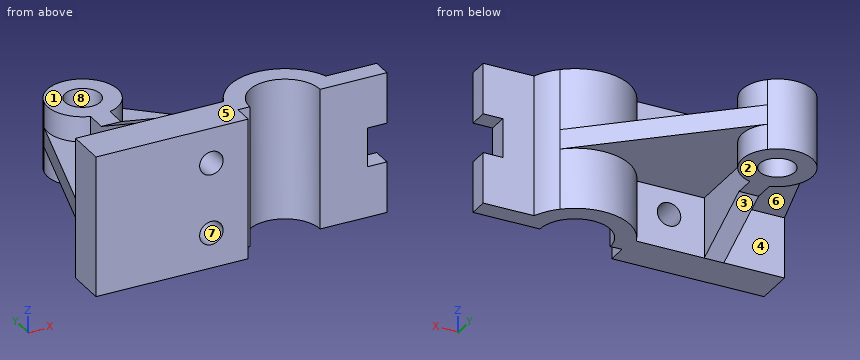
```python
from build123d import *

# Parameters (mm, degrees)
BOSS_EXTRUDE1_DEPTH      = 36
BOSS_EXTRUDE1_DEPTH_BACK = 36
BOSS_EXTRUDE2_DEPTH      = 18
BOSS_EXTRUDE2_DEPTH_BACK = 18
SKETCH2_3_R              = 9
BOSS_EXTRUDE3_DEPTH      = 5
BOSS_EXTRUDE3_DEPTH_BACK = 5
SKETCH2_4_W              = 5
SKETCH2_4_H              = 34
SKETCH3_W                = 10
SKETCH3_H                = 20
CUT_EXTRUDE1_DEPTH       = 178.234308191
RIB1_START               = -5
RIB1_DEPTH               = 10
SKETCH5_R                = 6
CUT_EXTRUDE2_DEPTH       = 178.234308191


# Read off the part's stored shape, not the designer's step: Rib1
with BuildPart() as part:
    # Sketch2 → Boss-Extrude1 (new, two sides: drawn at the far end of the back side and taken through both)
    with BuildSketch(Plane.XY.offset(-BOSS_EXTRUDE1_DEPTH_BACK)):
        with BuildLine():
            Line((0, 20), (0, 0))
            Line((0, 0), (77.846606339, 0))
            Line((77.846606339, 0), (77.846606339, 10))
            Line((77.846606339, 10), (83.846606339, 10))
            ThreePointArc((83.846606339, 10), (101.846606339, 28), (119.846606339, 10))
            Line((119.846606339, 10), (154, 10))
            Line((154, 10), (154, 20))
            Line((154, 20), (128, 20))
            ThreePointArc((128, 20), (124.887273582, 25.909985951), (120.463315732, 30.914543538))
            ThreePointArc((120.463315732, 30.914543538), (95.214697292, 37.203267863), (75.693212678, 20))
            Line((75.693212678, 20), (41, 20))
            Line((41, 20), (31, 20))
            Line((31, 20), (0, 20))
        make_face()
    extrude(amount=BOSS_EXTRUDE1_DEPTH + BOSS_EXTRUDE1_DEPTH_BACK)



with BuildPart() as body_2:
    # Sketch2<3> → Boss-Extrude2 (new, two sides: drawn at the far end of the back side and taken through both)
    with BuildSketch(Plane.XY.offset(-BOSS_EXTRUDE2_DEPTH_BACK)):
        with BuildLine():
            ThreePointArc((47.96788461, 95.445063703), (30.929004292, 99.270929405), (18.663131241, 86.840762505))
            ThreePointArc((18.663131241, 86.840762505), (20.277580459, 73.236123929), (31, 64.708383534))
            Line((31, 64.708383534), (31, 54))
            Line((31, 54), (41, 54))
            Line((41, 54), (41, 64.708383534))
            ThreePointArc((41, 64.708383534), (53.55457644, 78.020446505), (47.96788461, 95.445063703))
        make_face()
        with Locations((36, 82)):
            Circle(SKETCH2_3_R, mode=Mode.SUBTRACT)
    extrude(amount=BOSS_EXTRUDE2_DEPTH + BOSS_EXTRUDE2_DEPTH_BACK)


with BuildPart() as part_1:
    add(part.part)

    add(body_2.part)  # Boss-Extrude3 merges body 2
    # Sketch2<4> → Boss-Extrude3 (add, two sides: drawn at the far end of the back side and taken through both)
    with BuildSketch(Plane.XY.offset(-BOSS_EXTRUDE3_DEPTH_BACK)):
        with BuildLine():
            Line((120.463315732, 30.914543538), (47.96788461, 95.445063703))
            ThreePointArc((47.96788461, 95.445063703), (53.55457644, 78.020446505), (41, 64.708383534))
            Line((41, 64.708383534), (41, 54))
            Line((41, 54), (41, 20))
            Line((41, 20), (75.693212678, 20))
            ThreePointArc((75.693212678, 20), (95.214697292, 37.203267863), (120.463315732, 30.914543538))
        make_face()
        with Locations((33.5, 37)):
            Rectangle(SKETCH2_4_W, SKETCH2_4_H)
        with Locations((38.5, 37)):
            Rectangle(SKETCH2_4_W, SKETCH2_4_H)
        with BuildLine():
            Line((18.663131241, 86.840762505), (0, 20))
            Line((0, 20), (31, 20))
            Line((31, 20), (31, 54))
            Line((31, 54), (31, 64.708383534))
            ThreePointArc((31, 64.708383534), (20.277580459, 73.236123929), (18.663131241, 86.840762505))
        make_face()
    extrude(amount=BOSS_EXTRUDE3_DEPTH + BOSS_EXTRUDE3_DEPTH_BACK)

    # Sketch3 → Cut-Extrude1 (cut, through all)
    with BuildSketch(Plane(origin=(0, 20, 0), x_dir=(1, 0, 0), z_dir=(0, 1, 0))):
        with Locations((149, 0)):
            Rectangle(SKETCH3_W, SKETCH3_H)
    extrude(amount=-CUT_EXTRUDE1_DEPTH, mode=Mode.SUBTRACT)

    # Rib1 outline → Rib1 (add)
    with BuildSketch(Plane.ZY.offset(-36).offset(RIB1_START)):
        Polygon((36, 20), (18, 54), (5, 54), (5, 20), align=None)
    rib1 = extrude(amount=RIB1_DEPTH)

    # Mirror1: Rib1 across plane
    add(rib1.mirror(Plane.XY))

    # Sketch5 → Cut-Extrude2 (cut, through all)
    with BuildSketch(Plane(origin=(0, 20, 0), x_dir=(1, 0, 0), z_dir=(0, 1, 0))):
        with Locations(Location((59, -18, 0), (0, 0, 180))):
            Circle(SKETCH5_R)
        with Locations((59, 18)):
            Circle(SKETCH5_R)
    extrude(amount=-CUT_EXTRUDE2_DEPTH, mode=Mode.SUBTRACT)


solid = part_1.part
```
Part model, mm, in its own coordinate system. Face numbers are marked on the shaded views. A direction names the side the tool comes from. Coordinates: 2 decimals unless noted, no trailing zeros. Order: outer loops, then holes, each group sorted by start corner. A loop starts at its lowest first (then second) coordinate and runs counter-clockwise, first axis right, second up. Notation, with made-up numbers: (-27.75, -4) -> (16.25, -4) arc R12 cw to (16.25, 6) -> close; hole circle Ø6 at (68.5, 74.25). An arc over 180 degrees is marked (long way). Put each result on its own line as item: value. Start each with the question number.
(1) Probe line 1 along Z through (x, y) = (59, 8); line 2 along X through (y, z) = (13.75, -18); line 3 along Y through (x, z) = (36, -3). List the from-to ranges inside material, lowest first. Write a range as [from, to].
(2) Pin check, flat tips, straight feed: pin 1 Ø1.5 at (x, z) = (94, -6.5) entering from +Y; pin 2 Ø11 at (y, z) = (5.5, 11.5) entering from +X; pin 3 Ø21 at (x, z) = (136, -9) entering from +Y; pin 4 Ø18 at (x, y) = (37, 73.5) entering from -Z. Stop position of each tip, or through.
(3) Band-saw the part on C-C (y = 22). Give the cut face in (x, z), then the cut area to 3 significant figures.
(4) Mould opens along Z. For the marked faces 5, 6, 7 and 8 say: pulls with the +Z half, pulls with the -Z half, needs draft (parallel to the pull), parting line crosses it, or undercut.
(5) Band-saw the part on D-D (x = 36). Give the cut face in (y, z), then the cut area to 3 significant figures.
(6) Band-saw the part on A-A (x = 58). Give the cut face in (y, z).
(7) Which spindle directions (+Z, -Z, +X, -X, +Y, -Y) get a long thin tool onto all of the face, cutting with end or side? Do the marked faces 1, 2, 3 and 4. Say none if no direction does.
(8) Band-saw the part on B-B (z = 21). Give the cut face in (x, y).
Determined:
1. line 1: z = [-36, -24], [-12, 12], [24, 36]
1. line 2: x = [0, 53], [65, 84.24], [119.45, 154]
1. line 3: y = [0, 73], [91, 100]
2. pin 1: stops at y = 37.09
2. pin 2: stops at x = 154
2. pin 3: stops at y = 24.98
2. pin 4: stops at z = -18
3. outline: (0.56, -5) -> (31, -5) -> (31, -34.94) -> (41, -34.94) -> (41, -5) -> (76.55, -5) -> (76.55, -36) -> (88.43, -36) -> (88.43, 36) -> (76.55, 36) -> (76.55, 5) -> (41, 5) -> (41, 34.94) -> (31, 34.94) -> (31, 5) -> (0.56, 5) -> close; (115.26, -36) -> (127.14, -36) -> (127.14, 36) -> (115.26, 36) -> close
3. area: 3,070 mm²
4. face 5: pulls with the +Z half
4. face 6: pulls with the -Z half
4. face 7: undercut
4. face 8: needs draft
5. outline: (0, -36) -> (20, -36) -> (54, -18) -> (73, -18) -> (73, 18) -> (54, 18) -> (20, 36) -> (0, 36) -> close; (91, -18) -> (100, -18) -> (100, 18) -> (91, 18) -> close
5. area: 4,280 mm²
6. outline: (0, -36) -> (20, -36) -> (20, -23.92) -> (0, -23.92) -> close; (0, -12.08) -> (20, -12.08) -> (20, -5) -> (86.52, -5) -> (86.52, 5) -> (20, 5) -> (20, 12.08) -> (0, 12.08) -> close; (0, 23.92) -> (20, 23.92) -> (20, 36) -> (0, 36) -> close
7. face 1: +Z, +X, -X, +Y
7. face 2: -Z, +X, -X, +Y
7. face 3: -Z, -X, +Y
7. face 4: -Z, -X
8. outline: (0, 0) -> (53.8, 0) -> (53.8, 20) -> (41, 20) -> (41, 48.33) -> (31, 48.33) -> (31, 20) -> (0, 20) -> close; (64.2, 0) -> (77.85, 0) -> (77.85, 10) -> (83.85, 10) arc R18 cw to (119.85, 10) -> (154, 10) -> (154, 20) -> (128, 20) arc R28 ccw to (75.69, 20) -> (64.2, 20) -> close
